from build123d import *

# Parameters (mm, degrees)
SKETCH1_W               = 25.4
SKETCH1_H               = 29.275000124
BOSS_EXTRUDE1_DEPTH     = 3
SKETCH2_W               = 6.35
SKETCH2_H               = 3
BOSS_EXTRUDE2_DEPTH     = 6
LPATTERN1_COUNT         = 2
LPATTERN1_PITCH         = 12.7
MIRROR1_COPY_1_SKETCH_W = 6.35
MIRROR1_COPY_1_SKETCH_H = 3
MIRROR1_COPY_1_DEPTH    = 6
CUT_EXTRUDE1_DEPTH      = 25.417133509
CUT_EXTRUDE1_DEPTH_BACK = 25.417133509
FILLET1_R               = 2.54
FILLET2_R               = 2.54


with BuildPart() as part:
    # Sketch1 → Boss-Extrude1 (new body)
    with BuildSketch(Plane(origin=(0, 0, 0), x_dir=(1, 0, 0), z_dir=(0, 1, 0))):
        Rectangle(SKETCH1_W, SKETCH1_H)
    extrude(amount=BOSS_EXTRUDE1_DEPTH)

    # Sketch2 → Boss-Extrude2 (add)
    with BuildSketch(Plane.XY.offset(14.637500062)):
        with Locations((-6.35, 1.5)):
            Rectangle(SKETCH2_W, SKETCH2_H)
    boss_extrude2 = extrude(amount=BOSS_EXTRUDE2_DEPTH)

    # LPattern1: Boss-Extrude2 ×2
    with Locations(*[(i * LPATTERN1_PITCH, 0, 0) for i in range(1, LPATTERN1_COUNT)]):
        add(boss_extrude2)

    # Mirror1: Boss-Extrude2 across plane
    add(boss_extrude2.mirror(Plane.XY))

    # Mirror1 copy 1 sketch → Mirror1 copy 1 (add)
    with BuildSketch(Plane(origin=(12.7, 0, -14.637500062), x_dir=(1, 0, 0), z_dir=(0, 0, -1))):
        with Locations((-6.35, -1.5)):
            Rectangle(MIRROR1_COPY_1_SKETCH_W, MIRROR1_COPY_1_SKETCH_H)
    extrude(amount=MIRROR1_COPY_1_DEPTH)

    # Sketch4 → Cut-Extrude1 (cut, two sides: drawn at the far end of the back side and taken through both)
    with BuildSketch(Plane(origin=(0, 3, 0), x_dir=(1, 0, 0), z_dir=(0, 1, 0)).offset(-CUT_EXTRUDE1_DEPTH_BACK)):
        Polygon((7.460937373, -11.462500062), (-9.525, 8.978582163), (-9.525, -11.462500062), align=None)
        Polygon((9.525, 11.462500062), (-7.460937373, 11.462500062), (9.525, -8.978582163), align=None)
    extrude(amount=CUT_EXTRUDE1_DEPTH + CUT_EXTRUDE1_DEPTH_BACK, mode=Mode.SUBTRACT)

    # Fillet1
    fillet1_edges = [part.edges().sort_by_distance(p)[0] for p in [
        (-7.460937373, 1.5, -11.462500062),
        (9.525, 1.5, -11.462500062),
        (9.525, 1.5, 8.978582163),
        (-9.525, 1.5, -8.978582163),
        (7.460937373, 1.5, 11.462500062),
        (-9.525, 1.5, 11.462500062),
    ]]
    fillet(fillet1_edges, radius=FILLET1_R)

    # Fillet2
    fillet2_edges = [part.edges().sort_by_distance(p)[0] for p in [
        (-9.525, 1.5, 20.637500062),
        (-3.175, 1.5, 20.637500062),
        (3.175, 1.5, 20.637500062),
        (9.525, 1.5, 20.637500062),
        (-9.525, 1.5, -20.637500062),
        (-3.175, 1.5, -20.637500062),
        (3.175, 1.5, -20.637500062),
        (9.525, 1.5, -20.637500062),
    ]]
    fillet(fillet2_edges, radius=FILLET2_R)


solid = part.part
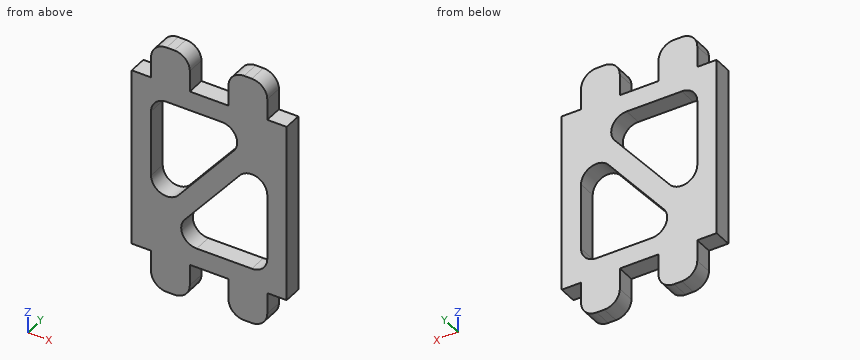
Build history of the part. All positions in model axes, mm. Round coordinates to 2 decimals unless told otherwise and drop trailing zeros. Write each loop counter-clockwise with the first axis right and the second up, starting at its lowest first coordinate (ties: lowest second). Pieces come first, ordered by that corner, then holes. Notation, with made-up numbers: (-39, 41.25) -> (-8, 41.25) arc R22 cw to (-8, 48.25) -> close; hole circle Ø8 at (42, 57). An arc over 180 degrees is marked (long way). Use one line per item in the form item = value.
Q1. Drill centre lines: L1, parallel to X at y = 1.05, z = -17 (3 decimals); L2, parallel to X at y = 2.7, z = 1 (3 decimals); L3, parallel to Z at x = 5.5, y = 1.2. Where is each one in solid material? Low to high.
Conclusion:
L1 = -9.525 to -3.175, 3.175 to 9.525
L2 = -12.7 to -9.525, -1.233 to 2.895, 9.525 to 12.7
L3 = -20.63 to -11.46, 4.01 to 20.63
Q2. Band-saw the part on D-D, the plane x = 10.25. Write the cut outline in (y, z).
Conclusion:
outline = (0, -14.64) -> (3, -14.64) -> (3, 14.64) -> (0, 14.64) -> close
Q3. Band-saw the part on C-C, the plane z = -1.5. Write the cut outline in (x, y) (3 decimals).
Conclusion:
outline = (-12.7, 0) -> (-9.525, 0) -> (-9.525, 3) -> (-12.7, 3) -> close; (-3.311, 0) -> (0.818, 0) -> (0.818, 3) -> (-3.311, 3) -> close; (9.525, 0) -> (12.7, 0) -> (12.7, 3) -> (9.525, 3) -> close
Q4. Drop flat-ended pins along their axis: P1, Ø0.9, axis at x = 11.5, y = 2, coming from the +Z side; P2, Ø2, axis at x = 6.5, z = 1, coming from the -Y side; P3, Ø1.5, axis at y = 1, z = 16, coming from the +X side (3 decimals); P4, Ø1.5, axis at y = 1, z = -16, coming from the -X side (3 decimals). Give the stop position or say it passes through.
Conclusion:
P1 = 14.64
P2 = through
P3 = 9.525
P4 = -9.525
Q5. Band-saw the part on B-B, the plane x = -1.25. Write the cut outline in (y, z).
Conclusion:
outline = (0, -14.64) -> (3, -14.64) -> (3, -11.46) -> (0, -11.46) -> close; (0, -3.99) -> (3, -3.99) -> (3, 0.98) -> (0, 0.98) -> close; (0, 11.46) -> (3, 11.46) -> (3, 14.64) -> (0, 14.64) -> close
Q6. Band-saw the part on A-A, the plane z = 17.5. Write the cut outline in (x, y) (3 decimals).
Conclusion:
outline = (-9.525, 0) -> (-3.175, 0) -> (-3.175, 3) -> (-9.525, 3) -> close; (3.175, 0) -> (9.525, 0) -> (9.525, 3) -> (3.175, 3) -> close
